from build123d import *

# Parameters (mm, degrees)
F0_W     = 260
F0_H     = 230
F1_DEPTH = 26
F2_W     = 20
F2_H     = 115
F3_DEPTH = 30
F4_W     = 25
F4_H     = 50
F5_DEPTH = 40


with BuildPart() as f1:
    # F0 (on Right) → F1 (new body)
    with BuildSketch(Plane.YZ):
        Rectangle(F0_W, F0_H)
    extrude(amount=F1_DEPTH)

    # F2 (on face) → F3 (cut)
    with BuildSketch(Plane.YZ.offset(26)):
        with Locations((0, 57.5)):
            Rectangle(F2_W, F2_H)
    extrude(amount=-F3_DEPTH, mode=Mode.SUBTRACT)

    # F4 (on face) → F5 (join)
    with BuildSketch(Plane.XY.offset(115)):
        with Locations((38.5, 35)):
            Rectangle(F4_W, F4_H)
    extrude(amount=-F5_DEPTH)


solid = f1.part
Design review of the part built by this model. Coordinates are the model's own, in mm. A direction names the side the tool comes from. Round coordinates to 2 decimals unless told otherwise and drop trailing zeros. Loops run counter-clockwise (first coordinate to the right, second up) from the corner with the lowest first, then second, coordinate; pieces in that order, holes last. Notation, with made-up numbers: (24.25, 4.25) -> (34.25, 4.25) arc R14 cw to (34.25, 29.25) -> close; hole circle Ø7 at (-11.5, 1.5). An arc over 180 degrees is marked (long way). Use one line per item in the form item = value. Start each with the question number.
Q1. We need section D-D on y = -72. Give the boundary of the cut face in (x, z).
Q2. For pin 1 Ø1.5 at (y, z) = (-15.5, 62.5) entering from -X; pin 2 Ø12.5 at (x, y) = (33.5, 40.5) entering from -Z; pin 3 Ø7.5 at (x, z) = (37, 98) entering from +Y; pin 4 Ø12 at (x, z) = (36, -10.5) entering from -Y, all flat-tipped, find the tip position at first contact; note any pin that passes through.
Q3. Machinability: for faces 4 (the face through (13, -2, -115)), 5 (the face through (38, 35, 75)), 6 (the face through (13, -10, 57)), which of the approach directions +Z, -Z, +X, -X, +Y, -Y give a long, thin tool a straight path to every point of the face, cutting with its end or side? Answer none if there is none.
Q4. We need section A-A on z = 4. Give the boundary of the cut face in (x, y), then the cut area to 3 significant figures.
Q5. Wall thickness on line 1 along Y through (x, z) = (14, 62); line 2 along X through (y, z) = (79, 43.5); line 3 along Z through (x, y) = (24.5, 0): over which ranges is each line inside the solid? List them lowest first. Write a range as [from, to].
Q6. We need section B-B on x = 9. Give the boundary of the cut face in (y, z).
Q7. We need section C-C on z = 92.5. Give the boundary of the cut face in (x, y), then the cut area to 3 significant figures.
Q8. Draft analysis for pull direction Y (two halves, no side actions). For faces 1 (the face through (0, -2, -24)), 2 (the face through (13, 0, 0)), 3 (the face through (38, 60, 95)), state which applies: +Y half, -Y half, draft (parallel to the pull), parting line (faces both ways), or undercut.
Calculated:
q1.outline = (0, -115) -> (26, -115) -> (26, 115) -> (0, 115) -> close
q2.pin_1 = 0
q2.pin_2 = 75
q2.pin_3 = 60
q2.pin_4 = through
q3.face_4 = -Z, +X, -X, +Y, -Y
q3.face_5 = -Z, +X, +Y, -Y
q3.face_6 = +Z, +X, -X
q4.outline = (0, -130) -> (26, -130) -> (26, -10) -> (0, -10) -> close; (0, 10) -> (26, 10) -> (26, 130) -> (0, 130) -> close
q4.area = 6,240 mm²
q5.line_1 = [-130, -10], [10, 130]
q5.line_2 = [0, 26]
q5.line_3 = [-115, 0]
q6.outline = (-130, -115) -> (130, -115) -> (130, 115) -> (10, 115) -> (10, 0) -> (-10, 0) -> (-10, 115) -> (-130, 115) -> close
q7.outline = (0, -130) -> (26, -130) -> (26, -10) -> (0, -10) -> close; (0, 10) -> (51, 10) -> (51, 60) -> (26, 60) -> (26, 130) -> (0, 130) -> close
q7.area = 7,490 mm²
q8.face_1 = draft
q8.face_2 = undercut
q8.face_3 = +Y half
